Autodesk Fusion 360 part; units mm, degrees
sketch "Sketch1" plane through (0, 0, 0) normal (0, 1, 0) x (1, 0, 0)
  line L0 (0, 0) -> (0, 50)
  line L1 (0, 50) -> (88, 50)
  line L2 (88, 50) -> (88, 0)
  line L3 (88, 0) -> (0, 0)
  dimension "d1" = 50
  dimension "d2" = 88
extrude "Extrude1" add sketch "Sketch1" along normal blind 18
sketch "Sketch2" plane through (0, 18, 0) normal (0, 1, 0) x (-1, 0, 0)
  line L0 (-88, 0) -> (-88, -50)
  line L1 (-88, -50) -> (0, -50)
  line L2 (0, -50) -> (0, 0)
  line L3 (0, 0) -> (-88, 0)
  line L4 (-38, 0) -> (-38, -28)
  line L5 (-38, -28) -> (0, -28)
  line L6 (0, -28) -> (0, -40)
  line L7 (0, -40) -> (-38, -40)
  line L8 (-38, -40) -> (-38, -50)
  line L9 (-38, -50) -> (-50, -50)
  line L10 (-50, -50) -> (-50, -40)
  line L11 (-50, -40) -> (-88, -40)
  line L12 (-88, -40) -> (-88, -28)
  line L13 (-50, -28) -> (-50, 0)
  line L14 (-38, 0) -> (-50, 0)
  line L15 (-50, -28) -> (-88, -28)
  line L16 (-50, 0) -> (-38, 0)
extrude "Extrude2" add sketch "Sketch2" along normal blind 38 contours L0 L1 L2 L3 L4 L5 L6 L7 L8 L9 L10 L11 L12 L13 L14 L15 L16
sketch "Sketch3" plane through (0, 0, 0) normal (0, 0, 1) x (1, 0, 0)
sketch "Sketch4" plane through (0, 0, 0) normal (0, 0, 1) x (1, 0, 0)
  line L0 (0, 0) -> (88, 0)
  line L1 (88, 0) -> (88, 18)
  line L2 (88, 18) -> (50, 18)
  line L3 (50, 18) -> (50, 56)
  line L4 (50, 56) -> (38, 56)
  line L5 (38, 56) -> (38, 18)
  line L6 (38, 18) -> (0, 18)
  line L7 (0, 18) -> (0, 0)
  line L8 (88, 0) -> (-2.3828, 0) construction
sketch "Sketch5" plane through (88, 0, 0) normal (1, 0, 0) x (0, 0, -1)
  line L0 (0, 0) -> (50, 0)
  line L1 (50, 0) -> (50, 18)
  line L2 (50, 18) -> (40, 18)
  line L3 (40, 18) -> (40, 56)
  line L4 (40, 56) -> (28, 56)
  line L5 (28, 56) -> (28, 18)
  line L6 (28, 18) -> (0, 18)
  line L7 (0, 18) -> (0, 0)
sketch "Sketch6" plane through (0, 0, 0) normal (0, 0, 1) x (1, 0, 0)
sketch "Sketch7" plane through (0, 0, 0) normal (0, 0, 1) x (1, 0, 0)
sketch "Sketch9" plane through (0, 0, 0) normal (0, 0, 1) x (1, 0, 0)
sketch "Sketch10" plane through (0, 56, 0) normal (0, 1, 0) x (-1, 0, 0)
  line L0 (-50, -28) -> (-88, -28)
  line L1 (-88, -28) -> (-88, -40)
  line L2 (-88, -40) -> (-50, -40)
  line L3 (-50, -40) -> (-50, -50)
  line L4 (-50, -50) -> (-38, -50)
  line L5 (-38, -50) -> (-38, -40)
  line L6 (-38, -40) -> (0, -40)
  line L7 (0, -40) -> (0, -28)
  line L8 (0, -28) -> (-38, -28)
  line L9 (-38, -28) -> (-38, 0)
  line L10 (-38, 0) -> (-50, 0)
  line L11 (-50, 0) -> (-50, -28)
sketch "Sketch11" plane through (0, 0, 0) normal (0, 0, 1) x (1, 0, 0)
ref_plane "WorkPlane1" through (88, 0, 0) normal (-0.5543, -0.5543, -0.6208) x (0.7071, -0.7071, 0)
sketch "Sketch12" plane through (88, 0, 0) normal (-0.5543, -0.5543, -0.6208) x (0.7071, -0.7071, 0)
  line L0 (-83.6898, 2.465) -> (-36.8291, -71.3922)
  line L1 (-36.8291, -71.3922) -> (9.1129, 2.465)
  line L2 (9.1129, 2.465) -> (-83.6898, 2.465)
extrude "Extrude3" cut sketch "Sketch12" against normal blind 15
Input: part model. Units: mm. Frame: model coordinates. A direction names the side the tool comes from. Give positions to 0.01 mm unless a question says otherwise; leave off trailing zeros. Order: outer loops, then holes, each group sorted by start corner. A loop starts at its lowest first (then second) coordinate and runs counter-clockwise, first axis right, second up. Notation, with made-up numbers: (47.5, 10.5) - (96.5, 10.5) arc R10 ccw to (96.5, 14.5) - close; hole circle Ø5 at (14.25, 44.5). An arc over 180 degrees is marked (long way). Answer as a JSON object with one key per item and string values. Group by question number.
Q1. Cut plane B-B, the plane y = 23.5. Output: boundary loops of the cut face in (x, z).
Q2. First-contact query: pin 1 Ø1.5 at (y, z) = (25.5, -15) entering from -X; pin 2 Ø14 at (y, z) = (34.5, -20) entering from +X; pin 3 Ø12 at (y, z) = (50, -36) entering from +X. Flat tips, straight axial feed; report the tip coordinate or a pass-through.
Q3. Line query: probe 1 along Y at (x, z) = (50.5, -9); probe 2 along Z at (x, y) = (20, 52); probe 3 along X at (y, z) = (44.5, -25). Output: solid intervals per line, ascending.
Q4. Cut plane C-C, the plane z = -42. Output: boundary loops of the cut face in (x, y), then the cut area to 3 significant figures.
Q5. Cut plane A-A, the plane x = 32. Output: boundary loops of the cut face in (y, z), then the cut area to 3 significant figures.
Q6. Set-up query: faces 1 (the face through (45, 14, 0)), 2 (the face through (65, 33, -28)), 3 (the face through (38, 37, -45)), 4 (the face through (19, 37, -28)), 5 (the face through (50, 37, -45)). Return all of +Z, -Z, +X, -X, +Y, -Y with unobstructed straight access to the full face (end or side cutting, diameter ignored); none if empty.
Q7. Cut plane D-D, the plane y = 42. Output: boundary loops of the cut face in (x, z).
Results:
{
 "1": {"outline": "(0, -40) - (38, -40) - (38, -50) - (50, -50) - (50, -40) - (88, -40) - (88, -28) - (50, -28) - (50, 0) - (38, 0) - (38, -28) - (0, -28) - close"},
 "2": {"pin 1": "x = 38", "pin 2": "x = 50", "pin 3": "x = 87.27"},
 "3": {"probe 1": "0 to 18", "probe 2": "-40 to -28", "probe 3": "38 to 50"},
 "4": {"outline": "(0, 0) - (88, 0) - (88, 18) - (50, 18) - (50, 56) - (38, 56) - (38, 18) - (0, 18) - close", "area": "2,040 mm^2"},
 "5": {"outline": "(0, -50) - (18, -50) - (18, -40) - (56, -40) - (56, -28) - (18, -28) - (18, 0) - (0, 0) - close", "area": "1,360 mm^2"},
 "6": {"face 1": "+Z, +X, -X, +Y, -Y", "face 2": "+Z, +X, +Y", "face 3": "-Z, -X, +Y", "face 4": "+Z, -X, +Y", "face 5": "-Z, +X, +Y"},
 "7": {"outline": "(0, -40) - (38, -40) - (38, -50) - (50, -50) - (50, -40) - (88, -40) - (88, -37.5) - (77.36, -28) - (50, -28) - (50, -3.57) - (46, 0) - (38, 0) - (38, -28) - (0, -28) - close"}
}
